The listing builds one solid part. Answer for the finished solid, in the listing's coordinates (mm). A direction names the side the tool comes from. Coordinates: 2 decimals unless noted, no trailing zeros. Order: outer loops, then holes, each group sorted by start corner. A loop starts at its lowest first (then second) coordinate and runs counter-clockwise, first axis right, second up.
Autodesk Fusion 360 part; units mm, degrees
sketch "スケッチ1" plane through (0, 0, 0) normal (0, 1, 0) x (1, 0, 0)
  line L0 (10, -10) -> (-10, -10)
  line L1 (-10, -10) -> (-10, 10)
  line L2 (-10, 10) -> (10, 10)
  line L3 (10, 10) -> (10, -10)
  line L4 (10, -10) -> (-10, 10) construction
  line L5 (-10, -10) -> (10, 10) construction
  dimension "d1" = 20
  dimension "d2" = 20
extrude "押し出し1" add sketch "スケッチ1" along normal blind 2
sketch "スケッチ2" plane through (0, 2, 0) normal (0, 1, 0) x (-1, 0, 0)
  line L0 (-10, -10) -> (10, -10)
  line L1 (10, -10) -> (10, 10)
  line L2 (10, 10) -> (-10, 10)
  line L3 (-10, 10) -> (-10, -10)
  line L4 (-7.5, 7.5) -> (7.5, 7.5)
  line L5 (7.5, 7.5) -> (7.5, -7.5)
  line L6 (7.5, -7.5) -> (-7.5, -7.5)
  line L7 (-7.5, -7.5) -> (-7.5, 7.5)
  line L8 (-7.5, 7.5) -> (7.5, -7.5) construction
  line L9 (7.5, 7.5) -> (-7.5, -7.5) construction
  dimension "d5" = 15
  dimension "d6" = 15
extrude "押し出し2" add sketch "スケッチ2" along normal blind 58 contours L4 L5 L6 L7
sketch "スケッチ3" plane through (0, 60, 0) normal (0, 1, 0) x (-1, 0, 0)
  line L0 (-7.5, -7.5) -> (7.5, -7.5)
  line L1 (7.5, -7.5) -> (7.5, 7.5)
  line L2 (7.5, 7.5) -> (-7.5, 7.5)
  line L3 (-7.5, 7.5) -> (-7.5, -7.5)
  line L4 (4.5, -7.5) -> (4.5, 4.5)
  line L5 (4.5, 4.5) -> (-7.5, 4.5)
  dimension "d9" = 3
  dimension "d10" = 3
extrude "押し出し3" add sketch "スケッチ3" along normal blind 10 contours L0 L1 L2 L3 L4 L5
move_face "面をオフセット1" offset 5 1 faces at (10, 0.6667, -3.3333)
move_face "面をオフセット2" offset 5 1 faces at (6.6667, 1.3333, -10)
(1) Find section B-B on x = -3.25. Determine the outline of the cut face in (y, z), then the cut area to 3 significant figures.
(2) Find section D-D on z = 2.5. Determine the outline of the cut face in (x, y).
(3) Find section C-C on y = 10.5. Determine the outline of the cut face in (x, z).
(4) A tool of negligible diameter and unlimited length cuts with its end or side. For faces 1 (the flat face through (7.5, 36, 0)), 2 (the flat face through (2, 60, -1)), 3 (the flat face through (0, 36, -7.5)), from which of +Z, -Z, +X, -X, +Y, -Y can it reach the whole face along a straight path? Write none if from no direction.
(5) Find section A-A on z = 5.5. Determine the outline of the cut face in (x, y), then the cut area to 3 significant figures.
(6) Find the intervals of material crossed by probe 1 along X at (y, z) = (52.5, 3.5); probe 2 along Y at (x, z) = (12.5, 6.5), in increasing order.
(7) Given pin 1 Ø5 at (y, z) = (63, 0.5) entering from +X; pin 2 Ø4 at (x, y) = (9, 47.5) entering from -Z; pin 3 Ø7.5 at (y, z) = (35, 0.5) entering from +X, each flat-ended and moving along its own axis, determine where each tip first touches the part or whether it passes through.
Resolved:
1. outline: (0, -15) - (2, -15) - (2, -7.5) - (60, -7.5) - (60, 4.5) - (70, 4.5) - (70, 7.5) - (2, 7.5) - (2, 10) - (0, 10) - close
1. area: 950 mm2
2. outline: (-10, 0) - (15, 0) - (15, 2) - (7.5, 2) - (7.5, 60) - (-4.5, 60) - (-4.5, 70) - (-7.5, 70) - (-7.5, 2) - (-10, 2) - close
3. outline: (-7.5, -7.5) - (7.5, -7.5) - (7.5, 7.5) - (-7.5, 7.5) - close
4. face 1: +Z, -Z, +X, +Y
4. face 2: -Z, +X, +Y
4. face 3: -Z, +X, -X, +Y
5. outline: (-10, 0) - (15, 0) - (15, 2) - (7.5, 2) - (7.5, 70) - (-7.5, 70) - (-7.5, 2) - (-10, 2) - close
5. area: 1,070 mm2
6. probe 1: x = -7.5 to 7.5
6. probe 2: y = 0 to 2
7. pin 1: stops at x = -4.5
7. pin 2: stops at z = -7.5
7. pin 3: stops at x = 7.5
